Check sheet for the modelled part. Datum: model origin and axes. Units: mm. A direction names the side the tool comes from. Round coordinates to 2 decimals unless told otherwise and drop trailing zeros. Order: outer loops, then holes, each group sorted by start corner. A loop starts at its lowest first (then second) coordinate and runs counter-clockwise, first axis right, second up.
(1) Sectioned sample at B-B, the plane x = 0. Enter the section's corners in (y, z).
(2) Mould release check, pull along X, two halves, no side actions. Record for faces 3 (the cylindrical face through (95.38, 30.04, 17.26)), 4 (the flat face through (-1, -21, 0)), 5 (the cylindrical face through (-56.582, -31.992, 32.605)), 6 (the cylindrical face through (-2.17, -9.76, 20.28)): released by +X, released by -X, zero draft, split by the parting line, or undercut.
(3) Depth check by flat-ended pin: pin 1 (15 mm diameter, centred on x = -41, y = -17, fed in from +Z); pin 2 (10 mm diameter, centred on x = 43, z = 26.5, fed in from +Y); pin 3 (8 mm diameter, centred on y = -16, z = 31.5, fed in from +X). Enter the tip coordinate at first touch or a pass-through.
(4) Tool access check on faces 1 (the flat face through (-1, -20, 40)), 2 (the cylindrical face through (-30.152, -17.772, 32.605)). Record the directions out of +Z, -Z, +X, -X, +Y, -Y that give a thin tool (end or side, any length) a straight path to the whole face; none if there is none.
(5) Sectioned sample at A-A, the plane y = 0. Enter the section's corners in (x, z).
(6) Sectioned sample at C-C, the plane z = 7. Enter the section's corners in (x, y).
(7) Thickness scan on probe 1 along Y at (x, z) = (0, 11); probe 2 along Y at (x, z) = (0, 30); probe 3 along Y at (x, z) = (-11.5, 22.5). Record the ranges inside material, lowest first.
```python
from build123d import *

# Parameters (mm, degrees)
SKETCH1_R           = 100
BOSS_EXTRUDE1_DEPTH = 40
CUT_EXTRUDE2_DEPTH  = 20
FILLET1_R           = 5
CHAMFER1_SIZE       = 5
SKETCH6_R           = 10
CUT_EXTRUDE3_DEPTH  = 147.969384635


with BuildPart() as part:
    # Sketch1 → Boss-Extrude1 (new body)
    with BuildSketch(Plane.XY):
        Circle(SKETCH1_R)
    extrude(amount=BOSS_EXTRUDE1_DEPTH)

    # Sketch5 → Cut-Extrude2 (cut)
    with BuildSketch(Plane.XY.offset(40)):
        with BuildLine():
            ThreePointArc((39, 52), (0, 65), (-39, 52))
            ThreePointArc((-39, 52), (-42, 31), (-21, 28))
            ThreePointArc((-21, 28), (0, 35), (21, 28))
            ThreePointArc((21, 28), (42, 31), (39, 52))
        make_face()
        with BuildLine():
            ThreePointArc((25.533320997, -59.774990748), (56.291651246, -32.5), (64.533320997, 7.774990748))
            ThreePointArc((64.533320997, 7.774990748), (47.846787517, 20.873066959), (34.748711306, 4.186533479))
            ThreePointArc((34.748711306, 4.186533479), (30.310889132, -17.5), (13.748711306, -32.186533479))
            ThreePointArc((13.748711306, -32.186533479), (5.846787517, -51.873066959), (25.533320997, -59.774990748))
        make_face()
        with BuildLine():
            ThreePointArc((-64.533320997, 7.774990748), (-56.291651246, -32.5), (-25.533320997, -59.774990748))
            ThreePointArc((-25.533320997, -59.774990748), (-5.846787517, -51.873066959), (-13.748711306, -32.186533479))
            ThreePointArc((-13.748711306, -32.186533479), (-30.310889132, -17.5), (-34.748711306, 4.186533479))
            ThreePointArc((-34.748711306, 4.186533479), (-47.846787517, 20.873066959), (-64.533320997, 7.774990748))
        make_face()
    extrude(amount=-CUT_EXTRUDE2_DEPTH, mode=Mode.SUBTRACT)

    # Fillet1
    fillet1_edges = [part.edges().sort_by_distance(p)[0] for p in [
        (-100, 0, 40),
    ]]
    fillet(fillet1_edges, radius=FILLET1_R)

    # Chamfer1
    chamfer1_edges = [part.edges().sort_by_distance(p)[0] for p in [
        (42, 31, 20),
        (0, 35, 20),
        (-42, 31, 20),
        (0, 65, 20),
        (5.846787517, -51.873066959, 20),
        (30.310889132, -17.5, 20),
        (47.846787517, 20.873066959, 20),
        (56.291651246, -32.5, 20),
        (-47.846787517, 20.873066959, 20),
        (-30.310889132, -17.5, 20),
        (-5.846787517, -51.873066959, 20),
        (-56.291651246, -32.5, 20),
    ]]
    chamfer(chamfer1_edges, length=CHAMFER1_SIZE)

    # Sketch6 → Cut-Extrude3 (cut, through all)
    with BuildSketch(Plane.XY.offset(40)):
        Circle(SKETCH6_R)
    extrude(amount=-CUT_EXTRUDE3_DEPTH, mode=Mode.SUBTRACT)


solid = part.part
```
Derived:
1. outline: (-100, 0) - (-10, 0) - (-10, 40) - (-95, 40) arc R5 ccw to (-100, 35) - close; (10, 0) - (100, 0) - (100, 35) arc R5 ccw to (95, 40) - (65, 40) - (65, 25) - (60, 20) - (40, 20) - (35, 25) - (35, 40) - (10, 40) - close
2. face 3: split by the parting line
2. face 4: zero draft
2. face 5: undercut
2. face 6: undercut
3. pin 1: stops at z = 23.12
3. pin 2: stops at y = 92.5
3. pin 3: stops at x = 99.28
4. face 1: +Z, +X, -X, +Y, -Y
4. face 2: +Z
5. outline: (-100, 0) - (-10, 0) - (-10, 40) - (-35, 40) - (-35, 25) - (-40, 20) - (-60, 20) - (-65, 25) - (-65, 40) - (-95, 40) arc R5 ccw to (-100, 35) - close; (10, 0) - (100, 0) - (100, 35) arc R5 ccw to (95, 40) - (65, 40) - (65, 25) - (60, 20) - (40, 20) - (35, 25) - (35, 40) - (10, 40) - close
6. outline: circle Ø200 at (0, 0); hole circle Ø20 at (0, 0)
7. probe 1: y = -100 to -10, 10 to 100
7. probe 2: y = -100 to -10, 10 to 35, 65 to 100
7. probe 3: y = -99.34 to -55.47, -36.5 to 35.69, 61.43 to 99.34
